from build123d import *

# Parameters (mm, degrees)
SKETCH1_W           = 180
SKETCH1_H           = 80
SKETCH1_R           = 23.75
BOSS_EXTRUDE1_DEPTH = 3
SKETCH2_W           = 6.4
SKETCH2_H           = 6.4
SKETCH2_W_2         = 6.402436435
CUT_EXTRUDE1_DEPTH  = 99.534258002
CUT_EXTRUDE2_DEPTH  = 3
SKETCH4_R           = 1.6
CUT_EXTRUDE3_DEPTH  = 3
SKETCH7_R           = 3.1
CUT_EXTRUDE4_DEPTH  = 3
FILLET1_R           = 10
FILLET2_R           = 15
FILLET3_R           = 10
FILLET4_R           = 1


with BuildPart() as part:
    # Sketch1 → Boss-Extrude1 (new body)
    with BuildSketch(Plane.XY):
        Rectangle(SKETCH1_W, SKETCH1_H)
        with Locations((55, 5)):
            Circle(SKETCH1_R, mode=Mode.SUBTRACT)
        with Locations((-55, 5)):
            Circle(SKETCH1_R, mode=Mode.SUBTRACT)
    extrude(amount=BOSS_EXTRUDE1_DEPTH)

    # Sketch2 → Cut-Extrude1 (cut, through all)
    with BuildSketch(Plane.XY.offset(3)):
        with Locations((-61, -28)):
            Rectangle(SKETCH2_W, SKETCH2_H)
        with Locations((-48.976364432, -28)):
            Rectangle(SKETCH2_W_2, SKETCH2_H)
        with Locations((-22, -1)):
            Rectangle(SKETCH2_W, SKETCH2_H)
        with Locations((-22, 11)):
            Rectangle(SKETCH2_W, SKETCH2_H)
        with Locations((22, -1)):
            Rectangle(SKETCH2_W, SKETCH2_H)
        with Locations((22, 11)):
            Rectangle(SKETCH2_W, SKETCH2_H)
        with Locations((49, -28)):
            Rectangle(SKETCH2_W, SKETCH2_H)
        with Locations((61, -28)):
            Rectangle(SKETCH2_W, SKETCH2_H)
    extrude(amount=-CUT_EXTRUDE1_DEPTH, mode=Mode.SUBTRACT)

    # Sketch3 → Cut-Extrude2 (cut)
    with BuildSketch(Plane.XY.offset(3)):
        Polygon((-21, -40), (-15, -34), (15, -34), (21, -40), align=None)
    extrude(amount=-CUT_EXTRUDE2_DEPTH, mode=Mode.SUBTRACT)

    # Sketch4 → Cut-Extrude3 (cut)
    with BuildSketch(Plane.XY.offset(3)):
        with Locations((-78.5, 28)):
            Circle(SKETCH4_R)
        with Locations((-31.545874822, 28)):
            Circle(SKETCH4_R)
        with Locations((-31.5, -18)):
            Circle(SKETCH4_R)
        with Locations((-78.5, -18)):
            Circle(SKETCH4_R)
        with Locations(Location((31.5, -18, 0), (0, 0, 180))):
            Circle(SKETCH4_R)
        with Locations(Location((31.545874822, 28, 0), (0, 0, 180))):
            Circle(SKETCH4_R)
        with Locations(Location((78.5, 28, 0), (0, 0, 180))):
            Circle(SKETCH4_R)
        with Locations(Location((78.5, -18, 0), (0, 0, 180))):
            Circle(SKETCH4_R)
    extrude(amount=-CUT_EXTRUDE3_DEPTH, mode=Mode.SUBTRACT)

    # Sketch7 → Cut-Extrude4 (cut)
    with BuildSketch(Plane.XY.offset(3)):
        Circle(SKETCH7_R)
        with Locations((0, 20)):
            Circle(SKETCH7_R)
    extrude(amount=-CUT_EXTRUDE4_DEPTH, mode=Mode.SUBTRACT)

    # Fillet1
    fillet1_edges = [part.edges().sort_by_distance(p)[0] for p in [
        (-90, 40, 1.5),
        (90, 40, 1.5),
    ]]
    fillet(fillet1_edges, radius=FILLET1_R)

    # Fillet2
    fillet2_edges = [part.edges().sort_by_distance(p)[0] for p in [
        (90, -40, 1.5),
        (-90, -40, 1.5),
    ]]
    fillet(fillet2_edges, radius=FILLET2_R)

    # Fillet3
    fillet3_edges = [part.edges().sort_by_distance(p)[0] for p in [
        (-15, -34, 1.5),
        (15, -34, 1.5),
        (21, -40, 1.5),
        (-21, -40, 1.5),
    ]]
    fillet(fillet3_edges, radius=FILLET3_R)

    # Fillet4
    fillet4_edges = [part.edges().sort_by_distance(p)[0] for p in [
        (45.8, -31.2, 1.5),
        (45.8, -24.8, 1.5),
        (52.2, -24.8, 1.5),
        (52.2, -31.2, 1.5),
        (57.8, -31.2, 1.5),
        (57.8, -24.8, 1.5),
        (64.2, -24.8, 1.5),
        (64.2, -31.2, 1.5),
        (-64.2, -24.8, 1.5),
        (-57.8, -24.8, 1.5),
        (-57.8, -31.2, 1.5),
        (-64.2, -31.2, 1.5),
        (-52.177582649, -31.2, 1.5),
        (-52.177582649, -24.8, 1.5),
        (-45.775146214, -24.8, 1.5),
        (-45.775146214, -31.2, 1.5),
        (-25.2, -4.2, 1.5),
        (-25.2, 2.2, 1.5),
        (-18.8, 2.2, 1.5),
        (-18.8, -4.2, 1.5),
        (-25.2, 7.8, 1.5),
        (-25.2, 14.2, 1.5),
        (-18.8, 14.2, 1.5),
        (-18.8, 7.8, 1.5),
        (18.8, -4.2, 1.5),
        (18.8, 2.2, 1.5),
        (25.2, 2.2, 1.5),
        (25.2, -4.2, 1.5),
        (18.8, 7.8, 1.5),
        (18.8, 14.2, 1.5),
        (25.2, 14.2, 1.5),
        (25.2, 7.8, 1.5),
    ]]
    fillet(fillet4_edges, radius=FILLET4_R)


solid = part.part
CAD build for the part. Positions are in the model's coordinates, mm. A direction names the side the tool comes from. Round coordinates to 2 decimals unless told otherwise and drop trailing zeros. Order: outer loops, then holes, each group sorted by start corner. A loop starts at its lowest first (then second) coordinate and runs counter-clockwise, first axis right, second up. Notation, with made-up numbers: (84.25, 41) -> (114.25, 41) arc R27 ccw to (114.25, 61) -> close; hole circle Ø5 at (-29.75, 88). An arc over 180 degrees is marked (long way). Write each question's results on one line, items separated by ' | '.
1. Cut at D-D (z = 1.7). Count the separate pieces of the cut face and the enclosed holes in it, plus the area to 3 significant figures.
Findings below:
separate pieces: 1 | enclosed holes: 20 | area: 10,100 mm²
2. Cut at C-C (x = 0). Give the cut face in (y, z), plus the area to 3 significant figures.
Findings below:
outline: (-34, 0) -> (-3.1, 0) -> (-3.1, 3) -> (-34, 3) -> close; (3.1, 0) -> (16.9, 0) -> (16.9, 3) -> (3.1, 3) -> close; (23.1, 0) -> (40, 0) -> (40, 3) -> (23.1, 3) -> close | area: 185 mm²
3. Flat gauge pins, fed straight in: P1, Ø0.9, axis at x = -22.5, z = 2, coming from the -Y side; P2, Ø1.5, axis at y = -27, z = 1.5, coming from the +X side; P3, Ø1.5, axis at y = -28, z = 1, coming from the -X side. Where does each tip first touch, or does it go through?
Findings below:
P1: stops at y = -39.76 | P2: stops at x = 89.95 | P3: stops at x = -89.83
4. Cut at B-B (y = 5). Give the cut face in (x, z), plus the area to 3 significant figures.
Findings below:
outline: (-90, 0) -> (-78.75, 0) -> (-78.75, 3) -> (-90, 3) -> close; (-31.25, 0) -> (31.25, 0) -> (31.25, 3) -> (-31.25, 3) -> close; (78.75, 0) -> (90, 0) -> (90, 3) -> (78.75, 3) -> close | area: 255 mm²
5. Pull direction Y, two halves, no side cores. Call faces 1 (the face through (-52.178, -28, 2)), 2 (the face through (90, 2, 1)), 3 (the face through (14.63, -34.74, 1.48)): pulls with the +Y half, pulls with the -Y half, needs draft (parallel to the pull), parting line crosses it, or undercut.
Findings below:
face 1: undercut | face 2: needs draft | face 3: pulls with the -Y half
6. 3-axis set-ups, long thin cutter, end or side, ignore diameter. For faces 4 (the face through (0, -34, 2)), 5 (the face through (-1, -8, 3)), 6 (the face through (18.8, -1, 2)): which of +Z, -Z, +X, -X, +Y, -Y reach the whole face in a straight line?
Findings below:
face 4: +Z, -Z, -Y | face 5: +Z, +X, -X, +Y, -Y | face 6: +Z, -Z
7. Cut at A-A (x = -55). Give the cut face in (y, z), plus the area to 3 significant figures.
Findings below:
outline: (-40, 0) -> (-18.75, 0) -> (-18.75, 3) -> (-40, 3) -> close; (28.75, 0) -> (40, 0) -> (40, 3) -> (28.75, 3) -> close | area: 97.5 mm²
8. Wall check: line 1 along Y through (x, z) = (0, 2.3); line 2 along Y through (x, z) = (-55.5, 0.2); line 3 along X through (y, z) = (-25, 2.4). Give the ranges that are in metal, low to high. Write a range as [from, to].
Findings below:
line 1: y = [-34, -3.1], [3.1, 16.9], [23.1, 40] | line 2: y = [-40, -18.74], [28.74, 40] | line 3: x = [-90, -63.8], [-58.2, -51.78], [-46.18, 46.2], [51.8, 58.2], [63.8, 90]
